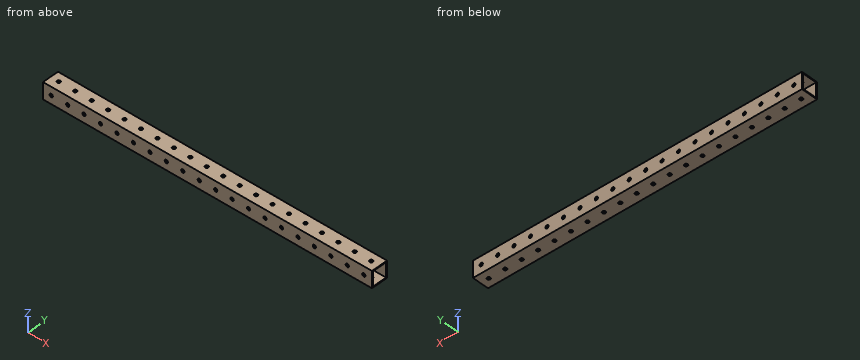
from build123d import *

# Parameters (mm, degrees)
SKETCH1_W             = 25.4
SKETCH1_H             = 25.4
SKETCH1_W_2           = 22.225
SKETCH1_H_2           = 22.225
BOSS_EXTRUDE1_DEPTH   = 254
SKETCH3_W             = 2.4892
SKETCH3_H             = 25.4
SKETCH3_AT_POINT_2_W  = 2.4892
SKETCH3_AT_POINT_2_H  = 25.4
LPATTERN1_START       = -12.7
LPATTERN1_OUTLINE_R   = 2.4892
LPATTERN1_DEPTH       = 25.4
LPATTERN1_2_OUTLINE_R = 2.4892
LPATTERN1_2_DEPTH     = 25.4


# Read off the part's stored shape, not the designer's step: LPattern1
with BuildPart() as part:
    # Sketch1 → Boss-Extrude1 (new, symmetric)
    with BuildSketch(Plane(origin=(0, 0, 0), x_dir=(0, 0, -1), z_dir=(1, 0, 0))):
        Rectangle(SKETCH1_W, SKETCH1_H)
        Rectangle(SKETCH1_W_2, SKETCH1_H_2, mode=Mode.SUBTRACT)
    extrude(amount=BOSS_EXTRUDE1_DEPTH, both=True)

    # Sketch3 → #9 (0.196) Diameter Hole1 (revolve, cut)
    with BuildSketch(Plane(origin=(241.3, 12.7, 0), x_dir=(0, 0, 1), z_dir=(1, 0, 0))):
        with Locations((1.2446, 12.7)):
            Rectangle(SKETCH3_W, SKETCH3_H)
    revolve(axis=Axis((241.3, 19.05, 0), (0, -1, 0)), mode=Mode.SUBTRACT)

    # Sketch3 at point 2 (carried to point 2, square into its face) → #9 (0.196) Diameter Hole1 at 2 (revolve, cut)
    with BuildSketch(Plane(origin=(241.3, 0, 12.7), x_dir=(0, -1, 0), z_dir=(1, 0, 0))):
        with Locations((1.2446, 12.7)):
            Rectangle(SKETCH3_AT_POINT_2_W, SKETCH3_AT_POINT_2_H)
    revolve(axis=Axis((241.3, 0, 19.05), (0, 0, -1)), mode=Mode.SUBTRACT)

    # LPattern1 outline → LPattern1 (cut)
    with BuildSketch(Plane.XY.offset(LPATTERN1_START)):
        with Locations((215.9, 0)):
            Circle(LPATTERN1_OUTLINE_R)
        with Locations((190.5, 0)):
            Circle(LPATTERN1_OUTLINE_R)
        with Locations((165.1, 0)):
            Circle(LPATTERN1_OUTLINE_R)
        with Locations((139.7, 0)):
            Circle(LPATTERN1_OUTLINE_R)
        with Locations((114.3, 0)):
            Circle(LPATTERN1_OUTLINE_R)
        with Locations((88.9, 0)):
            Circle(LPATTERN1_OUTLINE_R)
        with Locations((63.5, 0)):
            Circle(LPATTERN1_OUTLINE_R)
        with Locations((38.1, 0)):
            Circle(LPATTERN1_OUTLINE_R)
        with Locations((12.7, 0)):
            Circle(LPATTERN1_OUTLINE_R)
        with Locations((-12.7, 0)):
            Circle(LPATTERN1_OUTLINE_R)
        with Locations((-38.1, 0)):
            Circle(LPATTERN1_OUTLINE_R)
        with Locations((-63.5, 0)):
            Circle(LPATTERN1_OUTLINE_R)
        with Locations((-88.9, 0)):
            Circle(LPATTERN1_OUTLINE_R)
        with Locations((-114.3, 0)):
            Circle(LPATTERN1_OUTLINE_R)
        with Locations((-139.7, 0)):
            Circle(LPATTERN1_OUTLINE_R)
        with Locations((-165.1, 0)):
            Circle(LPATTERN1_OUTLINE_R)
        with Locations((-190.5, 0)):
            Circle(LPATTERN1_OUTLINE_R)
        with Locations((-215.9, 0)):
            Circle(LPATTERN1_OUTLINE_R)
        with Locations((-241.3, 0)):
            Circle(LPATTERN1_OUTLINE_R)
    extrude(amount=LPATTERN1_DEPTH, mode=Mode.SUBTRACT)

    # LPattern1 2 outline → LPattern1 2 (cut)
    with BuildSketch(Plane(origin=(0, 0, 0), x_dir=(1, 0, 0), z_dir=(0, 1, 0)).offset(LPATTERN1_START)):
        with Locations((215.9, 0)):
            Circle(LPATTERN1_2_OUTLINE_R)
        with Locations((190.5, 0)):
            Circle(LPATTERN1_2_OUTLINE_R)
        with Locations((165.1, 0)):
            Circle(LPATTERN1_2_OUTLINE_R)
        with Locations((139.7, 0)):
            Circle(LPATTERN1_2_OUTLINE_R)
        with Locations((114.3, 0)):
            Circle(LPATTERN1_2_OUTLINE_R)
        with Locations((88.9, 0)):
            Circle(LPATTERN1_2_OUTLINE_R)
        with Locations((63.5, 0)):
            Circle(LPATTERN1_2_OUTLINE_R)
        with Locations((38.1, 0)):
            Circle(LPATTERN1_2_OUTLINE_R)
        with Locations((12.7, 0)):
            Circle(LPATTERN1_2_OUTLINE_R)
        with Locations((-12.7, 0)):
            Circle(LPATTERN1_2_OUTLINE_R)
        with Locations((-38.1, 0)):
            Circle(LPATTERN1_2_OUTLINE_R)
        with Locations((-63.5, 0)):
            Circle(LPATTERN1_2_OUTLINE_R)
        with Locations((-88.9, 0)):
            Circle(LPATTERN1_2_OUTLINE_R)
        with Locations((-114.3, 0)):
            Circle(LPATTERN1_2_OUTLINE_R)
        with Locations((-139.7, 0)):
            Circle(LPATTERN1_2_OUTLINE_R)
        with Locations((-165.1, 0)):
            Circle(LPATTERN1_2_OUTLINE_R)
        with Locations((-190.5, 0)):
            Circle(LPATTERN1_2_OUTLINE_R)
        with Locations((-215.9, 0)):
            Circle(LPATTERN1_2_OUTLINE_R)
        with Locations((-241.3, 0)):
            Circle(LPATTERN1_2_OUTLINE_R)
    extrude(amount=LPATTERN1_2_DEPTH, mode=Mode.SUBTRACT)


solid = part.part
Here's how the part is built. I have some questions about the finished solid (model axes, mm). Give positions to 0.01 mm unless a question says otherwise; leave off trailing zeros. Write each loop counter-clockwise with the first axis right and the second up, starting at its lowest first coordinate (ties: lowest second). Pieces come first, ordered by that corner, then holes. Notation, with made-up numbers: (-13, 66) -> (7, 66) arc R20 ccw to (7, 79) -> close; hole circle Ø8 at (23.5, -12.75). An arc over 180 degrees is marked (long way). Use one line per item in the form item = value. Start each with the question number.
1. Imagine slicing it at A-A on z = -7.25. List the corners of the cut face in (x, y) for me.
2. Will these pins go through, and if not, where does the flat tip stop? pin 1 Ø8 at (x, z) = (38.1, 0) entering from -Y; pin 2 Ø3 at (x, z) = (190.5, 0) entering from -Y.
3. If I drill on L1, parallel to Z at x = 170, y = -5.25; L2, parallel to Y at x = -165.1, z = -12, over which ranges is the centre line in solid material (lowest first)?
4. Imagine slicing it at B-B on x = -5. List the corners of the cut face in (y, z) for me, plus the area to 3 significant figures.
Entries:
q1.outline = (-254, -12.7) -> (254, -12.7) -> (254, -11.11) -> (-254, -11.11) -> close; (-254, 11.11) -> (254, 11.11) -> (254, 12.7) -> (-254, 12.7) -> close
q2.pin_1 = -12.7
q2.pin_2 = through
q3.L1 = -12.7 to -11.11, 11.11 to 12.7
q3.L2 = -12.7 to -2.49, 2.49 to 12.7
q4.outline = (-12.7, -12.7) -> (12.7, -12.7) -> (12.7, 12.7) -> (-12.7, 12.7) -> close; hole (-11.11, -11.11) -> (11.11, -11.11) -> (11.11, 11.11) -> (-11.11, 11.11) -> close
q4.area = 151 mm²
